Input: part model. Units: mm. Frame: model coordinates. Face numbers are marked on the shaded views. A direction names the side the tool comes from. Give positions to 0.01 mm unless a question says otherwise; leave off trailing zeros. Loops run counter-clockwise (first coordinate to the right, second up) from the corner with the lowest first, then second, coordinate; pieces in that order, holes last. Notation, with made-up numbers: M 17,-39 L 55,-39 A26 cw 55,-15 Z; hole C 6.25,-10 d6. An arc over 180 degrees is marked long. One line per item, written item: value. Start each with the question number.
(1) Section A-A on z = -12. Output: boundary loops of the cut face in (x, y).
(2) Access query for the marked faces 1, 2 and 3. Directions: +Z, -Z, +X, -X, +Y, -Y. A direction counts if a zero-diameter tool reaches every point of the face in a straight line with its end or side. Return the directions, or none.
(3) Section B-B on x = 4.25. Output: boundary loops of the cut face in (y, z), plus the area to 3 significant figures.
(4) Section C-C on y = -103. Output: boundary loops of the cut face in (x, z), plus the area to 3 significant figures.
(5) Ray query, line 1 along Y through (x, z) = (0.25, -5.5); line 2 along Z through (x, y) = (-5.5, -106); line 3 along X through (y, z) = (-22.5, -20). Return the intervals inside material, ascending. Write a range as from..to.
(6) Pin query (flat end, axial travel): P1, Ø4.5, axis at x = -0.5, z = -9.5, coming from the -Y side; P2, Ø1.5, axis at x = -5, y = -99.5, coming from the +Z side; P3, Ø1.5, axis at y = -64, z = -19.5, coming from the +X side; P4, Ø2, axis at x = 3, y = -95.5, coming from the +Z side. Return the tip coordinate at first contact, or that it passes through.
```python
from build123d import *

# Parameters (mm, degrees)
BOX009_W                  = 94
BOX009_H                  = 15
BOX009_DEPTH              = 2
FILLET005_R               = 0.25
FILLET005_PLACEMENT_ANGLE = 90
BOX_W                     = 60
BOX_H                     = 17
BOX_DEPTH                 = 17
FILLET001_R               = 1
FILLET004_R               = 0.5
FILLET004_PLACEMENT_ANGLE = 90


with BuildPart() as obj1:
    # Box009 → Box009 (new body)
    with BuildSketch(Plane(origin=(-94, -6.5, -2), x_dir=(1, 0, 0), z_dir=(0, 0, 1))):
        with Locations((47, 7.5)):
            Rectangle(BOX009_W, BOX009_H)
    extrude(amount=BOX009_DEPTH)

    # Fillet005
    fillet005_edges = [obj1.edges().sort_by_distance(p)[0] for p in [
        (-94, -6.5, -1),
        (-94, 1, 0),
        (-94, 8.5, -1),
        (-94, 1, -2),
        (0, -6.5, -1),
        (0, 1, 0),
        (0, 8.5, -1),
        (0, 1, -2),
        (-47, -6.5, -2),
        (-47, -6.5, 0),
        (-47, 8.5, -2),
        (-47, 8.5, 0),
    ]]
    fillet(fillet005_edges, radius=FILLET005_R)


with BuildPart() as obj1_1:
    # Fillet005 placement: moved
    add(obj1.part.moved(Location((0, -16.75, -19.5))).rotate(Axis((0, -16.75, -19.5), (0, 0, 1)), FILLET005_PLACEMENT_ANGLE))


with BuildPart() as fusion034:
    # Box → Box (new body)
    with BuildSketch(Plane(origin=(0, -8.5, -17), x_dir=(1, 0, 0), z_dir=(0, 0, 1))):
        with Locations((30, 8.5)):
            Rectangle(BOX_W, BOX_H)
    extrude(amount=BOX_DEPTH)

    # Fillet001
    fillet001_edges = [fusion034.edges().sort_by_distance(p)[0] for p in [
        (0, -8.5, -8.5),
        (0, 8.5, -8.5),
        (60, -8.5, -8.5),
        (60, 8.5, -8.5),
    ]]
    fillet(fillet001_edges, radius=FILLET001_R)

    # Fillet004
    fillet004_edges = [fusion034.edges().sort_by_distance(p)[0] for p in [
        (0, 0, 0),
        (0, 0, -17),
        (30, -8.5, 0),
        (30, 8.5, 0),
        (60, 0, 0),
        (30, -8.5, -17),
        (30, 8.5, -17),
        (60, 0, -17),
    ]]
    fillet(fillet004_edges, radius=FILLET004_R)


with BuildPart() as fusion034_1:
    # Fillet004 placement: moved
    add(fusion034.part.moved(Location((0, -94.75, -2.5))).rotate(Axis((0, -94.75, -2.5), (0, 0, 1)), FILLET004_PLACEMENT_ANGLE))

    # Fusion034: union obj1
    add(obj1_1.part)


solid = fusion034_1.part
```
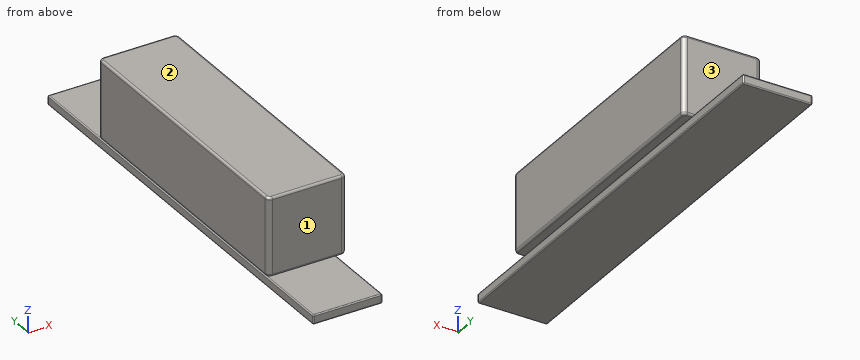
Output values:
1. outline: M -8.5,-93.75 A1 ccw -7.5,-94.75 L 7.5,-94.75 A1 ccw 8.5,-93.75 L 8.5,-35.75 A1 ccw 7.5,-34.75 L -7.5,-34.75 A1 ccw -8.5,-35.75 Z
2. face 1: +Z, +X, -X, -Y
2. face 2: +Z, +X, -X, +Y, -Y
2. face 3: +Z, +X, -X, +Y
3. outline: M -110.75,-21.25 A0.25 ccw -110.5,-21.5 L -17,-21.5 A0.25 ccw -16.75,-21.25 L -16.75,-19.75 A0.25 ccw -17,-19.5 L -35.25,-19.5 A0.5 ccw -34.75,-19 L -34.75,-3 A0.5 ccw -35.25,-2.5 L -94.25,-2.5 A0.5 ccw -94.75,-3 L -94.75,-19 A0.5 ccw -94.25,-19.5 L -110.5,-19.5 A0.25 ccw -110.75,-19.75 Z
3. area: 1,210 mm²
4. outline: M -8.5,-21.25 A0.25 ccw -8.25,-21.5 L 6.25,-21.5 A0.25 ccw 6.5,-21.25 L 6.5,-19.75 A0.25 ccw 6.25,-19.5 L -8.25,-19.5 A0.25 ccw -8.5,-19.75 Z
4. area: 29.9 mm²
5. line 1: y = -94.75..-34.75
5. line 2: z = -21.5..-19.5
5. line 3: x = -8.5..6.5
6. P1: stops at y = -94.75
6. P2: stops at z = -19.5
6. P3: stops at x = 8.5
6. P4: stops at z = -2.57
